Design review of the part built by this model. Coordinates are the model's own, in mm. Face numbers are marked on the shaded views. A direction names the side the tool comes from. Coordinates: 2 decimals unless noted, no trailing zeros. Write each loop counter-clockwise with the first axis right and the second up, starting at its lowest first coordinate (ties: lowest second). Pieces come first, ordered by that corner, then holes.
Q1. Take a section at B-B, the plane x = -29. Write out the cut boundary in (y, z), plus the area to 3 significant figures.
Q2. The part is to be moulded in two halves that separate along X. For the marked faces 4, 5 and 6, say which applies: released by +X, released by -X, zero draft, split by the parting line, or undercut.
Q3. Take a section at A-A, the plane y = 13. Write out the cut boundary in (x, z), plus the area to 3 significant figures.
Q4. For the marked faces 1, 2 and 3, list the 3-axis set-ups (+Z, -Z, +X, -X, +Y, -Y) from which the entire face can be reached by the end or side of a thin tool; tool diameter is ignored.
Q5. Take a section at C-C, the plane x = 50. Write out the cut boundary in (y, z), plus the area to 3 significant figures.
Q6. For L1, parallel to X at y = 7.75, z = 49.5; L2, parallel to Z at x = 58, y = 16.25; L3, parallel to Y at x = -34, z = 36, list the stretches that pass through material, from the lowest coordinate up.
Q7. Take a section at D-D, the plane z = 20.5. Write out the cut boundary in (x, y).
Q8. For pin 1 Ø5 at (x, y) = (46, 10) entering from +Z; pin 2 Ø6 at (x, z) = (6, 13) entering from +Y; pin 3 Ø4.5 at (y, z) = (8.5, 47.5) entering from +X; pin 4 Ø1.5 at (x, y) = (36, 3.5) entering from -Z, all flat-tipped, find the tip position at first contact; note any pin that passes through.
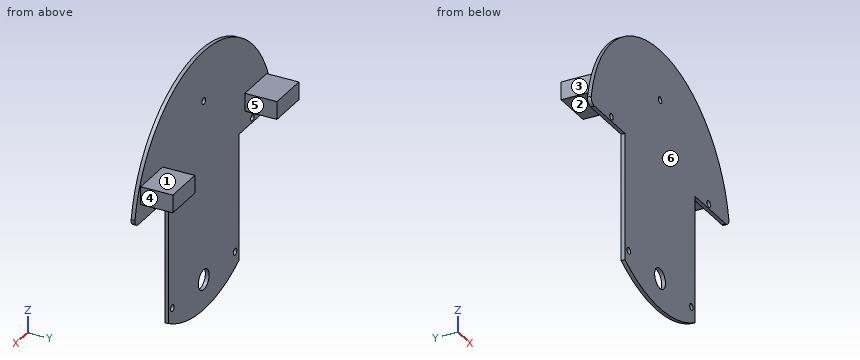
from build123d import *

# Parameters (mm, degrees)
SKETCH1_W           = 36
SKETCH1_H           = 20
BOSS_EXTRUDE1_DEPTH = 1.9
BOSS_EXTRUDE2_DEPTH = 1.9
CUT_EXTRUDE1_DEPTH  = 10
SKETCH5_R           = 5
CUT_EXTRUDE2_DEPTH  = 1.9
SKETCH6_R           = 1.6
CUT_EXTRUDE3_DEPTH  = 1.9
ESQUISSE1_W         = 20.3
ESQUISSE1_H         = 8.9
BOSS_EXTRU_1_DEPTH  = 16


with BuildPart() as part:
    # Sketch1 → Boss-Extrude1 (new body)
    with BuildSketch(Plane(origin=(0, 0, 0), x_dir=(1, 0, 0), z_dir=(0, 1, 0))):
        Rectangle(SKETCH1_W, SKETCH1_H)
    extrude(amount=BOSS_EXTRUDE1_DEPTH)

    # Sketch3 → Boss-Extrude2 (add)
    with BuildSketch(Plane.XZ):
        with BuildLine():
            Line((37.5, -26.725181376), (32.5, -26.725181376))
            Line((32.5, -26.725181376), (32.5, 33.274818624))
            Line((32.5, 33.274818624), (60.67226545, 33.274818624))
            ThreePointArc((60.67226545, 33.274818624), (62.960456011, 34.334668125), (63.631888155, 36.765362653))
            ThreePointArc((63.631888155, 36.765362653), (0, 90.718666019), (-63.631888155, 36.765362653))
            ThreePointArc((-63.631888155, 36.765362653), (-62.960456011, 34.334668125), (-60.67226545, 33.274818624))
            Line((-60.67226545, 33.274818624), (-32.5, 33.274818624))
            Line((-32.5, 33.274818624), (-32.5, -26.725181376))
            Line((-32.5, -26.725181376), (-37.5, -26.725181376))
            ThreePointArc((-37.5, -26.725181376), (0, -38.660459877), (37.5, -26.725181376))
        make_face()
    extrude(amount=-BOSS_EXTRUDE2_DEPTH)

    # Sketch4 → Cut-Extrude1 (cut)
    with BuildSketch(Plane(origin=(0, 1.9, 0), x_dir=(1, 0, 0), z_dir=(0, 1, 0))):
        Polygon((-32.5, 26.725181376), (-32.5, 34.194748576), (-40.442086395, 34.194748576), (-37.5, 26.725181376), align=None)
        Polygon((37.5, 26.725181376), (32.5, 26.725181376), (32.5, 34.194748576), (40.442086395, 34.194748576), align=None)
    extrude(amount=-CUT_EXTRUDE1_DEPTH, mode=Mode.SUBTRACT)

    # Sketch5 → Cut-Extrude2 (cut)
    with BuildSketch(Plane(origin=(0, 1.9, 0), x_dir=(1, 0, 0), z_dir=(0, 1, 0))):
        with Locations((0, 23.660459877)):
            Circle(SKETCH5_R)
    extrude(amount=-CUT_EXTRUDE2_DEPTH, mode=Mode.SUBTRACT)

    # Sketch6 → Cut-Extrude3 (cut)
    with BuildSketch(Plane(origin=(0, 1.9, 0), x_dir=(1, 0, 0), z_dir=(0, 1, 0))):
        with Locations((0, -65.718666019)):
            Circle(SKETCH6_R)
        with Locations((-45, -35.574302205)):
            Circle(SKETCH6_R)
        with Locations((45, -35.574302205)):
            Circle(SKETCH6_R)
        with Locations((-29, 23.804823691)):
            Circle(SKETCH6_R)
        with Locations((29, 23.804823691)):
            Circle(SKETCH6_R)
    extrude(amount=-CUT_EXTRUDE3_DEPTH, mode=Mode.SUBTRACT)

    # Esquisse1 → Boss.-Extru.1 (add)
    with BuildSketch(Plane(origin=(0, 1.9, 0), x_dir=(1, 0, 0), z_dir=(0, 1, 0))):
        with Locations((48.15, -46.724818624)):
            Rectangle(ESQUISSE1_W, ESQUISSE1_H)
        with Locations((-48.15, -46.724818624)):
            Rectangle(ESQUISSE1_W, ESQUISSE1_H)
    extrude(amount=BOSS_EXTRU_1_DEPTH)


solid = part.part
Responses:
1. outline: (0, -31.82) - (1.9, -31.82) - (1.9, -25.4) - (0, -25.4) - close; (0, -22.2) - (1.9, -22.2) - (1.9, 83.83) - (0, 83.83) - close
1. area: 214 mm2
2. face 4: released by +X
2. face 5: undercut
2. face 6: zero draft
3. outline: (-58.3, 42.27) - (-38, 42.27) - (-38, 51.17) - (-58.3, 51.17) - close; (38, 42.27) - (58.3, 42.27) - (58.3, 51.17) - (38, 51.17) - close
3. area: 361 mm2
4. face 1: +Z, +X, -X, +Y
4. face 2: -Z, +X, -X, +Y
4. face 3: +Z, -Z, -X, +Y
5. outline: (0, 33.27) - (1.9, 33.27) - (1.9, 42.27) - (17.9, 42.27) - (17.9, 51.17) - (1.9, 51.17) - (1.9, 66.96) - (0, 66.96) - close
5. area: 206 mm2
6. L1: x = -58.3 to -38, 38 to 58.3
6. L2: z = 42.27 to 51.17
6. L3: y = 0 to 1.9
7. outline: (-32.5, 0) - (32.5, 0) - (32.5, 1.9) - (-32.5, 1.9) - close
8. pin 1: stops at z = 51.17
8. pin 2: stops at y = 1.9
8. pin 3: stops at x = 58.3
8. pin 4: passes through
